from build123d import *

# Parameters (mm, degrees)
CROQUIS1_W              = 125
CROQUIS1_H              = 95
SALIENTE_EXTRUIR1_DEPTH = 11.2
CROQUIS2_W              = 58.3
CROQUIS2_H              = 91.2
CROQUIS2_W_2            = 6.4
CROQUIS2_H_2            = 6.4
CORTAR_EXTRUIR1_DEPTH   = 32.5
CORTAR_EXTRUIR2_DEPTH   = 4


with BuildPart() as part:
    # Croquis1 → Saliente-Extruir1 (new body)
    with BuildSketch(Plane.XY):
        with Locations((-11.370773818, -8.561811531)):
            Rectangle(CROQUIS1_W, CROQUIS1_H)
    extrude(amount=SALIENTE_EXTRUIR1_DEPTH)

    # Croquis2 → Cortar-Extruir1 (cut)
    with BuildSketch(Plane(origin=(0, 0, 0), x_dir=(-1, 0, 0), z_dir=(0, 0, -1))):
        with Locations((39.720773818, -8.711811531)):
            Rectangle(CROQUIS2_W, CROQUIS2_H)
        with Locations((-37.929226182, 25.738188469)):
            Rectangle(CROQUIS2_W_2, CROQUIS2_H_2)
        with Locations((-22.929226182, 25.738188469)):
            Rectangle(CROQUIS2_W_2, CROQUIS2_H_2)
        with Locations((-7.929226182, 25.738188469)):
            Rectangle(CROQUIS2_W_2, CROQUIS2_H_2)
        with Locations((-22.929226182, -8.561811531)):
            Rectangle(CROQUIS2_W_2, CROQUIS2_H_2)
        with Locations((-7.929226182, -8.561811531)):
            Rectangle(CROQUIS2_W_2, CROQUIS2_H_2)
        with Locations((-22.929226182, -42.861811531)):
            Rectangle(CROQUIS2_W_2, CROQUIS2_H_2)
        with Locations((-7.929226182, -42.861811531)):
            Rectangle(CROQUIS2_W_2, CROQUIS2_H_2)
        with Locations((-37.929226182, -8.561811531)):
            Rectangle(CROQUIS2_W_2, CROQUIS2_H_2)
        with Locations((-37.929226182, -42.861811531)):
            Rectangle(CROQUIS2_W_2, CROQUIS2_H_2)
    extrude(amount=-CORTAR_EXTRUIR1_DEPTH, mode=Mode.SUBTRACT)

    # Croquis3 → Cortar-Extruir2 (cut)
    with BuildSketch(Plane(origin=(0, 0, 0), x_dir=(-1, 0, 0), z_dir=(0, 0, -1))):
        Polygon((-39.429226182, 22.538188469), (-39.429226182, 17.538188469), (10.570773818, 17.538188469), (10.570773818, 20.538188469), (-6.429226182, 20.538188469), (-6.429226182, 22.538188469), (-9.429226182, 22.538188469), (-9.429226182, 20.538188469), (-21.429226182, 20.538188469), (-21.429226182, 22.538188469), (-24.429226182, 22.538188469), (-24.429226182, 20.538188469), (-36.429226182, 20.538188469), (-36.429226182, 22.538188469), align=None)
        Polygon((-9.429226182, -11.761811531), (-6.429226182, -11.761811531), (-6.429226182, -13.761811531), (10.570773818, -13.761811531), (10.570773818, -16.761811531), (-39.429226182, -16.761811531), (-39.429226182, -11.761811531), (-36.429226182, -11.761811531), (-36.429226182, -13.761811531), (-24.429226182, -13.761811531), (-24.429226182, -11.761811531), (-21.429226182, -11.761811531), (-21.429226182, -13.761811531), (-9.429226182, -13.761811531), align=None)
        Polygon((-9.429226182, -46.061811531), (-6.429226182, -46.061811531), (-6.429226182, -48.061811531), (10.570773818, -48.061811531), (10.570773818, -51.061811531), (-39.429226182, -51.061811531), (-39.429226182, -46.061811531), (-36.429226182, -46.061811531), (-36.429226182, -48.061811531), (-24.429226182, -48.061811531), (-24.429226182, -46.061811531), (-21.429226182, -46.061811531), (-21.429226182, -48.061811531), (-9.429226182, -48.061811531), align=None)
    extrude(amount=-CORTAR_EXTRUIR2_DEPTH, mode=Mode.SUBTRACT)


solid = part.part
The listing builds one solid part. Answer for the finished solid, in the listing's coordinates (mm). A direction names the side the tool comes from. Coordinates: 2 decimals unless noted, no trailing zeros. Loops run counter-clockwise (first coordinate to the right, second up) from the corner with the lowest first, then second, coordinate; pieces in that order, holes last. Notation, with made-up numbers: M 41,51 L 76,51 A28 ccw 76,82 Z; hole C 41.25,3.5 d5. An arc over 180 degrees is marked long. Answer in a Markdown table with one row per item.
1) Given pin 1 (2.5 mm diameter, centred on x = 24, y = 19, fed in from -Z), flat-ended and moving along its own axis, determine where the tip first touches the part or whether it passes through.
Answers below:
| item | result |
|---|---|
| pin 1 | z = 4 |
2) Find the intervals of material crossed by probe 1 along Y at (x, z) = (28, 1); probe 2 along Y at (x, z) = (41, 0.75); probe 3 along Y at (x, z) = (-49.5, 7), in increasing order.
Answers below:
| item | result |
|---|---|
| probe 1 | -56.06 to -51.06, -48.06 to -16.76, -13.76 to 17.54, 20.54 to 38.94 |
| probe 2 | -56.06 to -46.06, -39.66 to -11.76, -5.36 to 22.54, 28.94 to 38.94 |
| probe 3 | -56.06 to -54.31, 36.89 to 38.94 |
3) Find section C-C (y = -43.5). Determine the outline of the cut face in (x, z), then the cut area to 3 significant figures.
Answers below:
| item | result |
|---|---|
| outline | M -73.87,0 L -68.87,0 L -68.87,11.2 L -73.87,11.2 Z; M -10.57,0 L 4.73,0 L 4.73,11.2 L -10.57,11.2 Z; M 11.13,0 L 19.73,0 L 19.73,11.2 L 11.13,11.2 Z; M 26.13,0 L 34.73,0 L 34.73,11.2 L 26.13,11.2 Z; M 41.13,0 L 51.13,0 L 51.13,11.2 L 41.13,11.2 Z |
| area | 532 mm^2 |
4) Find section D-D (x = 33). Determine the outline of the cut face in (y, z), then the cut area to 3 significant figures.
Answers below:
| item | result |
|---|---|
| outline | M -56.06,0 L -51.06,0 L -51.06,4 L -48.06,4 L -48.06,0 L -16.76,0 L -16.76,4 L -13.76,4 L -13.76,0 L 17.54,0 L 17.54,4 L 20.54,4 L 20.54,0 L 38.94,0 L 38.94,11.2 L -56.06,11.2 Z |
| area | 1,030 mm^2 |
5) Find section A-A (y = -24). Determine the outline of the cut face in (x, z), then the cut area to 3 significant figures.
Answers below:
| item | result |
|---|---|
| outline | M -73.87,0 L -68.87,0 L -68.87,11.2 L -73.87,11.2 Z; M -10.57,0 L 51.13,0 L 51.13,11.2 L -10.57,11.2 Z |
| area | 747 mm^2 |
6) Determine the mould class of faces 3 (the flat face through (29, -8, 0)), 4 (the flat face through (23, -11.762, 7)) for opening direction X: released by +X, released by -X, zero draft, split by the parting line, or undercut.
Answers below:
| item | result |
|---|---|
| face 3 | zero draft |
| face 4 | undercut |
7) Find section B-B (x = -57). Determine the outline of the cut face in (y, z).
Answers below:
| item | result |
|---|---|
| outline | M -56.06,0 L -54.31,0 L -54.31,11.2 L -56.06,11.2 Z; M 36.89,0 L 38.94,0 L 38.94,11.2 L 36.89,11.2 Z |
8) Which of the six approach directions +Z, -Z, +X, -X, +Y, -Y give full straight-line access (tool end or side, diameter ignored) to faces 1 (the flat face through (23, 22.538, 7)), 2 (the flat face through (-2, 20.538, 2))?
Answers below:
| item | result |
|---|---|
| face 1 | +Z, -Z |
| face 2 | -Z |
